from build123d import *

# Parameters (mm, degrees)
F0_W     = 40
F0_H     = 50
F1_DEPTH = 11
F2_R     = 1.625
F3_DEPTH = 11.001
F4_W     = 25.5
F4_H     = 45
F5_DEPTH = 8
F6_R     = 5
F7_R     = 15
F8_DEPTH = 25


with BuildPart() as f1:
    # F0 (on Front) → F1 (new body)
    with BuildSketch(Plane.XZ):
        Rectangle(F0_W, F0_H)
    extrude(amount=F1_DEPTH)

    # F2 (on face) → F3 (cut, through all)
    with BuildSketch(Plane.XZ.offset(11)):
        with Locations((-16.125, 11)):
            Circle(F2_R)
        with Locations((16.125, 11)):
            Circle(F2_R)
    extrude(amount=-F3_DEPTH, mode=Mode.SUBTRACT)

    # F4 (on face) → F5 (cut)
    with BuildSketch(Plane(origin=(0, 0, 0), x_dir=(-1, 0, 0), z_dir=(0, 1, 0))):
        Rectangle(F4_W, F4_H)
    extrude(amount=-F5_DEPTH, mode=Mode.SUBTRACT)

    # F6
    f6_edges = [f1.edges().sort_by_distance(p)[0] for p in [
        (0, -8, 22.5),
    ]]
    fillet(f6_edges, radius=F6_R)

    # F7 (on face) → F8 (cut)
    with BuildSketch(Plane.XZ.offset(11)):
        with Locations((0, -5)):
            Circle(F7_R)
    extrude(amount=-F8_DEPTH, mode=Mode.SUBTRACT)


solid = f1.part
Verification items for the finished model (mm, model axes). A direction names the side the tool comes from. Coordinates: 2 decimals unless noted, no trailing zeros. Loops run counter-clockwise (first coordinate to the right, second up) from the corner with the lowest first, then second, coordinate; pieces in that order, holes last. Notation, with made-up numbers: (60.5, -24) -> (103.5, -24) arc R11 ccw to (103.5, -9) -> close; hole circle Ø3 at (58, 73.25). An arc over 180 degrees is marked (long way). Write each question's results on one line, items separated by ' | '.
Item 1: Section check D-D, the plane z = 11. Enter the section's corners in (x, y).
Found:
outline: (-20, -11) -> (-17.75, -11) -> (-17.75, 0) -> (-20, 0) -> close; (-14.5, -11) -> (14.5, -11) -> (14.5, 0) -> (12.75, 0) -> (12.75, -8) -> (-12.75, -8) -> (-12.75, 0) -> (-14.5, 0) -> close; (17.75, -11) -> (20, -11) -> (20, 0) -> (17.75, 0) -> close
Item 2: Gauge pin test, flat ends, axial feed: pin 1 (7.5 mm diameter, centred on x = 2, z = -16, fed in from +Y); pin 2 (10 mm diameter, centred on x = -13, z = 10.5, fed in from +Y); pin 3 (16 mm diameter, centred on x = 3, z = 12.5, fed in from +Y). Record the tip position at first contact, or that the pin passes through.
Found:
pin 1: passes through | pin 2: stops at y = 0 | pin 3: stops at y = -7
Item 3: Section check A-A, the plane z = -5. Enter the section's corners in (x, y).
Found:
outline: (-20, -11) -> (-15, -11) -> (-15, 0) -> (-20, 0) -> close; (15, -11) -> (20, -11) -> (20, 0) -> (15, 0) -> close
Item 4: Material ranges on L1, parallel to Z at x = -12.5, y = -2.25; L2, parallel to X at y = -1.75, z = -4.5; L3, parallel to X at y = -6, z = -17, recorded low to high.
Found:
L1: z = -25 to -22.5, 22.5 to 25 | L2: x = -20 to -14.99, 14.99 to 20 | L3: x = -20 to -12.75, 12.75 to 20
Item 5: Section check C-C, the plane x = 4. Enter the section's corners in (y, z), plus the area to 3 significant figures.
Found:
outline: (-11, -25) -> (0, -25) -> (0, -22.5) -> (-8, -22.5) -> (-8, -19.46) -> (-11, -19.46) -> close; (-11, 9.46) -> (-8, 9.46) -> (-8, 17.5) arc R5 cw to (-3, 22.5) -> (0, 22.5) -> (0, 25) -> (-11, 25) -> close | area: 109 mm2
Item 6: Mould release check, pull along X, two halves, no side actions. Record for faces 1 (the face through (-20, -5, 0)), 2 (the face through (20, -5, 0)), 3 (the face through (12.75, -4, 13)): +X half, -X half, draft (parallel to the pull), parting line (faces both ways), or undercut.
Found:
face 1: -X half | face 2: +X half | face 3: undercut
Item 7: Tool access check on faces 4 (the face through (-14, 0, 6)), 5 (the face through (0, -1, 22.5)). Record the directions out of +Z, -Z, +X, -X, +Y, -Y that give a thin tool (end or side, any length) a straight path to the whole face; none if there is none.
Found:
face 4: +Z, -Z, +X, -X, +Y | face 5: +Y
Item 8: Section check B-B, the plane y = -8.75. Enter the section's corners in (x, z) (3 decimals).
Found:
outline: (-20, -25) -> (20, -25) -> (20, 25) -> (-20, 25) -> close; hole circle Ø3.25 at (-16.125, 11); hole circle Ø30 at (0, -5); hole circle Ø3.25 at (16.125, 11)
